```python
from build123d import *

# Parameters (mm, degrees)
SKETCH1_R           = 52.5
SKETCH1_R_2         = 48.5
BOSS_EXTRUDE1_DEPTH = 100
SKETCH2_R           = 8
BOSS_EXTRUDE2_DEPTH = 100
BOSS_EXTRUDE3_START = -8
BOSS_EXTRUDE3_DEPTH = 4
BOSS_EXTRUDE4_START = -88
BOSS_EXTRUDE4_DEPTH = 4


with BuildPart() as part:
    # Sketch1 → Boss-Extrude1 (new body)
    with BuildSketch(Plane(origin=(0, 0, 0), x_dir=(1, 0, 0), z_dir=(0, 1, 0))):
        Circle(SKETCH1_R)
        Circle(SKETCH1_R_2, mode=Mode.SUBTRACT)
    extrude(amount=BOSS_EXTRUDE1_DEPTH)



with BuildPart() as body_2:
    # Sketch2 → Boss-Extrude2 (new body)
    with BuildSketch(Plane.XZ):
        Circle(SKETCH2_R)
        with BuildLine():
            ThreePointArc((3.5, -3.570714214), (-5, 0), (3.5, 3.570714214))
            Line((3.5, 3.570714214), (3.5, -3.570714214))
        make_face(mode=Mode.SUBTRACT)
    extrude(amount=-BOSS_EXTRUDE2_DEPTH)


with BuildPart() as part_1:
    add(part.part)

    add(body_2.part)  # Boss-Extrude3 merges body 2
    # Sketch2_3 → Boss-Extrude3 (add)
    with BuildSketch(Plane.XZ.offset(BOSS_EXTRUDE3_START)):
        with BuildLine():
            ThreePointArc((0, 8), (4.702282018, 6.472135955), (7.60845213, 2.472135955))
            Line((7.60845213, 2.472135955), (46.12624104, 14.987324227))
            ThreePointArc((46.12624104, 14.987324227), (28.507584736, 39.237324227), (0, 48.5))
            Line((0, 48.5), (0, 8))
        make_face()
        with BuildLine():
            Line((4.498612897, 20.291931451), (7.656121129, 34.53453068))
            ThreePointArc((7.656121129, 34.53453068), (9.081556968, 36.48129187), (11.479516965, 36.748750866))
            ThreePointArc((11.479516965, 36.748750866), (22.629732213, 31.147154283), (31.402773148, 22.273657954))
            ThreePointArc((31.402773148, 22.273657954), (31.889414918, 19.910413097), (30.4784189, 17.953160762))
            Line((30.4784189, 17.953160762), (17.908625798, 10.548986777))
            ThreePointArc((17.908625798, 10.548986777), (15.84479345, 10.183097432), (14.045152036, 11.257606507))
            ThreePointArc((14.045152036, 11.257606507), (10.580134541, 14.562305899), (6.366429359, 16.836525093))
            ThreePointArc((6.366429359, 16.836525093), (4.78839072, 18.216044222), (4.498612897, 20.291931451))
        make_face(mode=Mode.SUBTRACT)
        with BuildLine():
            Line((46.12624104, 14.987324227), (7.60845213, 2.472135955))
            ThreePointArc((7.60845213, 2.472135955), (7.901506725, 1.25147572), (8, 0))
            ThreePointArc((8, 0), (-5.656854249, -5.656854249), (0, 8))
            Line((0, 8), (0, 48.5))
            ThreePointArc((0, 48.5), (-34.294678888, -34.294678888), (48.5, 0))
            ThreePointArc((48.5, 0), (47.902884519, 7.587071554), (46.12624104, 14.987324227))
        make_face()
        with BuildLine():
            Line((8.287843762, -19.060735709), (14.104955724, -32.439177302))
            ThreePointArc((14.104955724, -32.439177302), (14.096031424, -34.851990353), (12.313249487, -36.477854749))
            ThreePointArc((12.313249487, -36.477854749), (0, -38.5), (-12.313249487, -36.477854749))
            ThreePointArc((-12.313249487, -36.477854749), (-14.096031424, -34.851990353), (-14.104955724, -32.439177302))
            Line((-14.104955724, -32.439177302), (-8.287843762, -19.060735709))
            ThreePointArc((-8.287843762, -19.060735709), (-6.83323268, -17.551634794), (-4.745711605, -17.363128214))
            ThreePointArc((-4.745711605, -17.363128214), (0, -18), (4.745711605, -17.363128214))
            ThreePointArc((4.745711605, -17.363128214), (6.83323268, -17.551634794), (8.287843762, -19.060735709))
        make_face(mode=Mode.SUBTRACT)
        with BuildLine():
            Line((-15.566752332, -13.772299075), (-26.492819932, -23.438867123))
            ThreePointArc((-26.492819932, -23.438867123), (-28.790299268, -24.175979847), (-30.887498112, -22.982873197))
            ThreePointArc((-30.887498112, -22.982873197), (-36.615675877, -11.897154283), (-38.497504807, 0.438319126))
            ThreePointArc((-38.497504807, 0.438319126), (-37.502125795, 2.636265233), (-35.21016198, 3.390352984))
            Line((-35.21016198, 3.390352984), (-20.688921471, 1.992116557))
            ThreePointArc((-20.688921471, 1.992116557), (-18.804181667, 1.075037038), (-17.979821767, -0.852061747))
            ThreePointArc((-17.979821767, -0.852061747), (-17.119017293, -5.562305899), (-15.046810695, -9.87894164))
            ThreePointArc((-15.046810695, -9.87894164), (-14.581011618, -11.922543898), (-15.566752332, -13.772299075))
        make_face(mode=Mode.SUBTRACT)
        with BuildLine():
            Line((20.688921471, 1.992116557), (35.21016198, 3.390352984))
            ThreePointArc((35.21016198, 3.390352984), (37.502125795, 2.636265233), (38.497504807, 0.438319126))
            ThreePointArc((38.497504807, 0.438319126), (36.615675877, -11.897154283), (30.887498112, -22.982873197))
            ThreePointArc((30.887498112, -22.982873197), (28.790299268, -24.175979847), (26.492819932, -23.438867123))
            Line((26.492819932, -23.438867123), (15.566752332, -13.772299075))
            ThreePointArc((15.566752332, -13.772299075), (14.581011618, -11.922543898), (15.046810695, -9.87894164))
            ThreePointArc((15.046810695, -9.87894164), (17.119017293, -5.562305899), (17.979821767, -0.852061747))
            ThreePointArc((17.979821767, -0.852061747), (18.804181667, 1.075037038), (20.688921471, 1.992116557))
        make_face(mode=Mode.SUBTRACT)
        with BuildLine():
            Line((-17.908625798, 10.548986777), (-30.4784189, 17.953160762))
            ThreePointArc((-30.4784189, 17.953160762), (-31.889414918, 19.910413097), (-31.402773148, 22.273657954))
            ThreePointArc((-31.402773148, 22.273657954), (-22.629732213, 31.147154283), (-11.479516965, 36.748750866))
            ThreePointArc((-11.479516965, 36.748750866), (-9.081556968, 36.48129187), (-7.656121129, 34.53453068))
            Line((-7.656121129, 34.53453068), (-4.498612897, 20.291931451))
            ThreePointArc((-4.498612897, 20.291931451), (-4.78839072, 18.216044222), (-6.366429359, 16.836525093))
            ThreePointArc((-6.366429359, 16.836525093), (-10.580134541, 14.562305899), (-14.045152036, 11.257606507))
            ThreePointArc((-14.045152036, 11.257606507), (-15.84479345, 10.183097432), (-17.908625798, 10.548986777))
        make_face(mode=Mode.SUBTRACT)
    extrude(amount=-BOSS_EXTRUDE3_DEPTH)

    # Sketch2_4 → Boss-Extrude4 (add)
    with BuildSketch(Plane.XZ.offset(BOSS_EXTRUDE4_START)):
        with BuildLine():
            Line((46.12624104, 14.987324227), (7.60845213, 2.472135955))
            ThreePointArc((7.60845213, 2.472135955), (7.901506725, 1.25147572), (8, 0))
            ThreePointArc((8, 0), (-5.656854249, -5.656854249), (0, 8))
            Line((0, 8), (0, 48.5))
            ThreePointArc((0, 48.5), (-34.294678888, -34.294678888), (48.5, 0))
            ThreePointArc((48.5, 0), (47.902884519, 7.587071554), (46.12624104, 14.987324227))
        make_face()
        with BuildLine():
            Line((8.287843762, -19.060735709), (14.104955724, -32.439177302))
            ThreePointArc((14.104955724, -32.439177302), (14.096031424, -34.851990353), (12.313249487, -36.477854749))
            ThreePointArc((12.313249487, -36.477854749), (0, -38.5), (-12.313249487, -36.477854749))
            ThreePointArc((-12.313249487, -36.477854749), (-14.096031424, -34.851990353), (-14.104955724, -32.439177302))
            Line((-14.104955724, -32.439177302), (-8.287843762, -19.060735709))
            ThreePointArc((-8.287843762, -19.060735709), (-6.83323268, -17.551634794), (-4.745711605, -17.363128214))
            ThreePointArc((-4.745711605, -17.363128214), (0, -18), (4.745711605, -17.363128214))
            ThreePointArc((4.745711605, -17.363128214), (6.83323268, -17.551634794), (8.287843762, -19.060735709))
        make_face(mode=Mode.SUBTRACT)
        with BuildLine():
            Line((-15.566752332, -13.772299075), (-26.492819932, -23.438867123))
            ThreePointArc((-26.492819932, -23.438867123), (-28.790299268, -24.175979847), (-30.887498112, -22.982873197))
            ThreePointArc((-30.887498112, -22.982873197), (-36.615675877, -11.897154283), (-38.497504807, 0.438319126))
            ThreePointArc((-38.497504807, 0.438319126), (-37.502125795, 2.636265233), (-35.21016198, 3.390352984))
            Line((-35.21016198, 3.390352984), (-20.688921471, 1.992116557))
            ThreePointArc((-20.688921471, 1.992116557), (-18.804181667, 1.075037038), (-17.979821767, -0.852061747))
            ThreePointArc((-17.979821767, -0.852061747), (-17.119017293, -5.562305899), (-15.046810695, -9.87894164))
            ThreePointArc((-15.046810695, -9.87894164), (-14.581011618, -11.922543898), (-15.566752332, -13.772299075))
        make_face(mode=Mode.SUBTRACT)
        with BuildLine():
            Line((20.688921471, 1.992116557), (35.21016198, 3.390352984))
            ThreePointArc((35.21016198, 3.390352984), (37.502125795, 2.636265233), (38.497504807, 0.438319126))
            ThreePointArc((38.497504807, 0.438319126), (36.615675877, -11.897154283), (30.887498112, -22.982873197))
            ThreePointArc((30.887498112, -22.982873197), (28.790299268, -24.175979847), (26.492819932, -23.438867123))
            Line((26.492819932, -23.438867123), (15.566752332, -13.772299075))
            ThreePointArc((15.566752332, -13.772299075), (14.581011618, -11.922543898), (15.046810695, -9.87894164))
            ThreePointArc((15.046810695, -9.87894164), (17.119017293, -5.562305899), (17.979821767, -0.852061747))
            ThreePointArc((17.979821767, -0.852061747), (18.804181667, 1.075037038), (20.688921471, 1.992116557))
        make_face(mode=Mode.SUBTRACT)
        with BuildLine():
            Line((-17.908625798, 10.548986777), (-30.4784189, 17.953160762))
            ThreePointArc((-30.4784189, 17.953160762), (-31.889414918, 19.910413097), (-31.402773148, 22.273657954))
            ThreePointArc((-31.402773148, 22.273657954), (-22.629732213, 31.147154283), (-11.479516965, 36.748750866))
            ThreePointArc((-11.479516965, 36.748750866), (-9.081556968, 36.48129187), (-7.656121129, 34.53453068))
            Line((-7.656121129, 34.53453068), (-4.498612897, 20.291931451))
            ThreePointArc((-4.498612897, 20.291931451), (-4.78839072, 18.216044222), (-6.366429359, 16.836525093))
            ThreePointArc((-6.366429359, 16.836525093), (-10.580134541, 14.562305899), (-14.045152036, 11.257606507))
            ThreePointArc((-14.045152036, 11.257606507), (-15.84479345, 10.183097432), (-17.908625798, 10.548986777))
        make_face(mode=Mode.SUBTRACT)
        with BuildLine():
            ThreePointArc((0, 8), (4.702282018, 6.472135955), (7.60845213, 2.472135955))
            Line((7.60845213, 2.472135955), (46.12624104, 14.987324227))
            ThreePointArc((46.12624104, 14.987324227), (28.507584736, 39.237324227), (0, 48.5))
            Line((0, 48.5), (0, 8))
        make_face()
        with BuildLine():
            Line((4.498612897, 20.291931451), (7.656121129, 34.53453068))
            ThreePointArc((7.656121129, 34.53453068), (9.081556968, 36.48129187), (11.479516965, 36.748750866))
            ThreePointArc((11.479516965, 36.748750866), (22.629732213, 31.147154283), (31.402773148, 22.273657954))
            ThreePointArc((31.402773148, 22.273657954), (31.889414918, 19.910413097), (30.4784189, 17.953160762))
            Line((30.4784189, 17.953160762), (17.908625798, 10.548986777))
            ThreePointArc((17.908625798, 10.548986777), (15.84479345, 10.183097432), (14.045152036, 11.257606507))
            ThreePointArc((14.045152036, 11.257606507), (10.580134541, 14.562305899), (6.366429359, 16.836525093))
            ThreePointArc((6.366429359, 16.836525093), (4.78839072, 18.216044222), (4.498612897, 20.291931451))
        make_face(mode=Mode.SUBTRACT)
    extrude(amount=-BOSS_EXTRUDE4_DEPTH)


solid = part_1.part
```
CAD build for the part. Positions are in the model's coordinates, mm. A direction names the side the tool comes from. Give positions to 0.01 mm unless a question says otherwise; leave off trailing zeros. Write each loop counter-clockwise with the first axis right and the second up, starting at its lowest first coordinate (ties: lowest second). Pieces come first, ordered by that corner, then holes. Notation, with made-up numbers: (26.5, 65.5) -> (71.5, 65.5) arc R16 ccw to (71.5, 70.5) -> close; hole circle Ø2 at (80.5, 73.5). An arc over 180 degrees is marked (long way). Write each question's results on one line, items separated by ' | '.
1. Wall check: probe 1 along X at (y, z) = (97.25, 0); probe 2 along Y at (x, z) = (23.5, 35.5); probe 3 along Z at (x, y) = (0, 2). Give the ranges that are in metal, low to high. Write a range as [from, to].
Geometry check:
probe 1: [-52.5, -48.5], [-8, -5], [3.5, 8], [48.5, 52.5] | probe 2: [8, 12], [88, 92] | probe 3: [-52.5, -48.5], [-8, -5], [5, 8], [48.5, 52.5]
2. Which spindle directions (+Z, -Z, +X, -X, +Y, -Y) get a long thin tool onto all of the face, cutting with end or side? Do faces 3 (the cylindrical face through (28.825, 89.972, -24.172)), 4 (the cylindrical face through (46.26, 95.94, -14.57)). Say none if no direction does.
Geometry check:
face 3: +Y, -Y | face 4: +Y
3. Two-plate mould, pull along Z, no slides. Class faces 1 (the cylindrical face through (-18.825, 9.972, 1.097)), 2 (the flat face through (-24.11, 89.97, 14.2)): pulls with the +Z half, pulls with the -Z half, needs draft (parallel to the pull), parting line crosses it, or undercut.
Geometry check:
face 1: undercut | face 2: undercut
4. Cut at A-A, the plane y = 82.5. Write the cut outline in (x, z).
Geometry check:
outline: circle Ø105 at (0, 0); circle Ø16 at (0, 0); hole circle Ø97 at (0, 0); hole (3.5, -3.57) -> (3.5, 3.57) arc R5 ccw (long way) to start
5. Drop flat-ended pins along their axis: P1, Ø5, axis at y = 54, z = -10.5, coming from the -X side; P2, Ø5, axis at y = 82.5, z = 34.5, coming from the -X side; P3, Ø2, axis at y = 59.5, z = -37.5, coming from the +X side. Give the stop position or say it passes through.
Geometry check:
P1: x = -51.89 | P2: x = -41.62 | P3: x = 37.74
6. Cut at C-C, the plane z = 39. Write the cut outline in (x, y).
Geometry check:
outline: (-35.15, 0) -> (-28.83, 0) -> (-28.83, 8) -> (28.83, 8) -> (28.83, 0) -> (35.15, 0) -> (35.15, 100) -> (28.83, 100) -> (28.83, 92) -> (-28.83, 92) -> (-28.83, 100) -> (-35.15, 100) -> close; hole (-28.83, 12) -> (28.83, 12) -> (28.83, 88) -> (-28.83, 88) -> close
7. Cut at B-B, the plane x = 0. Give the number of separate pieces and of enclosed holes in the cut face, then the cut area to 3 significant figures.
Geometry check:
separate pieces: 3 | enclosed holes: 1 | area: 1,880 mm²
